```python
from build123d import *

# Parameters (mm, degrees)
F1_DEPTH = 63.5
F0_W     = 25.4
F0_H     = 19.05
F0_H_2   = 4.7498
F0_H_3   = 4.7752
F2_DEPTH = 25.4


with BuildPart() as f1:
    # F0 (on Front) → F1 (new body, symmetric)
    with BuildSketch(Plane.XZ):
        Polygon((22.225, 9.525), (-41.275, 9.525), (-41.275, -9.525), (41.275, -9.525), (41.275, 9.525), align=None)
    extrude(amount=F1_DEPTH, both=True)

    # F0 (on Front) → F2 (join)
    with BuildSketch(Plane.XZ):
        with BuildLine():
            add(Edge.make_bspline(
                [(-41.275, 9.525), (-17.5234507769, 39.429217577), (10.7755595818, 66.2067756057), (57.15, 61.9252)],
                knots=[0, 0, 0, 0, 111.5045361635, 111.5045361635, 111.5045361635, 111.5045361635], degree=3))
            Line((-41.275, 9.525), (22.225, 9.525))
            Line((22.225, 9.525), (22.225, 27.0002))
            ThreePointArc((22.225, 27.0002), (32.4542956671, 51.6959043329), (57.15, 61.9252))
        make_face()
        Polygon((22.225, 9.525), (-41.275, 9.525), (-41.275, -9.525), (41.275, -9.525), (41.275, 9.525), align=None)
        with BuildLine():
            Line((22.225, 27.0002), (22.225, 9.525))
            Line((22.225, 9.525), (41.275, 9.525))
            Line((41.275, 9.525), (41.275, 27.0002))
            ThreePointArc((41.275, 27.0002), (45.9246798487, 38.2255201513), (57.15, 42.8752))
            Line((57.15, 42.8752), (60.325, 42.8752))
            Line((60.325, 42.8752), (60.325, 61.9252))
            Line((60.325, 61.9252), (57.15, 61.9252))
            ThreePointArc((57.15, 61.9252), (32.4542956671, 51.6959043329), (22.225, 27.0002))
        make_face()
        with Locations((73.025, 52.4002)):
            Rectangle(F0_W, F0_H)
        with Locations((73.025, 64.3001)):
            Rectangle(F0_W, F0_H_2)
        with Locations((73.025, 40.4876)):
            Rectangle(F0_W, F0_H_3)
        Polygon((85.725, 66.675), (85.725, 61.9252), (85.725, 42.8752), (85.725, 38.1), (111.125, 38.1), (111.125, 66.675), align=None)
    extrude(amount=F2_DEPTH)


solid = f1.part
```
Geometry check sheet. Reference: the model listing, model coordinates, mm. A direction names the side the tool comes from. Coordinates: 2 decimals unless noted, no trailing zeros. Order: outer loops, then holes, each group sorted by start corner. A loop starts at its lowest first (then second) coordinate and runs counter-clockwise, first axis right, second up. Notation, with made-up numbers: (-28.5, -33) - (29.5, -33) arc R14 cw to (29.5, -18) - close; hole circle Ø3 at (-26.75, 32). An arc over 180 degrees is marked (long way). Answer in a Markdown table with one row per item. Add a question column.
1. Draft check along X on faces 1 (the face through (-1, -63.5, 0)), 2 (the face through (45.8, -12.5, 38.1)), 3 (the face through (-41.275, 1, 0)), 4 (the face through (41.275, 1, 0)). Enter one of: +X half, -X half, draft (parallel to the pull), parting line (faces both ways), or undercut.
2. Gauge pin test, flat ends, axial feed: pin 1 Ø2.5 at (x, y) = (58.5, -13.5) entering from -Z; pin 2 Ø12 at (x, z) = (82, 37.5) entering from -Y; pin 3 Ø7.5 at (x, y) = (90.5, -17.5) entering from -Z. Record the tip position at first contact, or that the pin passes through.
3. Material ranges on L1, parallel to Y at x = 13, z = 18; L2, parallel to Z at x = 30, y = 9.5 (3 decimals); L3, parallel to Z at x = 66, y = -2 (3 decimals), recorded low to high. Write a range as [from, to].
4. Access from +Z, -Z, +X, -X, +Y, -Y to the whole of each face (thin tool, end or side, straight path). Record for faces 5 (the face through (1, 31, 9.525)), 6 (the face through (-1, 1, -9.525)), 7 (the face through (1, -45, 9.525)), 8 (the face through (60.325, -13, 40)), 9 (the face through (85, -13, 38.1)).
5. Section check B-B (z = 5.5). Enter the section's corners in (x, y) (3 decimals).
6. Section check A-A (x = 92). Enter the section's corners in (y, z) (3 decimals).
Data:
| question | item | result |
|---|---|---|
| 1 | face 1 | draft |
| 1 | face 2 | undercut |
| 1 | face 3 | -X half |
| 1 | face 4 | +X half |
| 2 | pin 1 | stops at z = 42.88 |
| 2 | pin 2 | stops at y = -25.4 |
| 2 | pin 3 | stops at z = 38.1 |
| 3 | L1 | y = [-25.4, 0] |
| 3 | L2 | z = [-9.525, 9.525] |
| 3 | L3 | z = [38.1, 66.675] |
| 4 | face 5 | +Z, +X, -X, +Y |
| 4 | face 6 | -Z, +X, -X, +Y, -Y |
| 4 | face 7 | +Z, +X, -X, -Y |
| 4 | face 8 | -Z, +Y, -Y |
| 4 | face 9 | -Z, +X, +Y, -Y |
| 5 | outline | (-41.275, -63.5) - (41.275, -63.5) - (41.275, 63.5) - (-41.275, 63.5) - close |
| 6 | outline | (-25.4, 38.1) - (0, 38.1) - (0, 66.675) - (-25.4, 66.675) - close |
